Autodesk Inventor part; units mm, degrees
ref_plane "YZ Plane" through (0, 0, 0) normal (1, 0, 0) x (0, 1, 0)
ref_plane "XZ Plane" through (0, 0, 0) normal (0, 1, 0) x (-1, 0, 0)
ref_plane "XY Plane" through (0, 0, 0) normal (0, 0, 1) x (1, 0, 0)
sketch "Sketch1" plane through (0, 0, 0) normal (0, 0, 1) x (1, 0, 0)
  line L0 (0, 0) -> (44, 0)
  line L1 (44, 0) -> (44, 10)
  line L2 (44, 10) -> (0, 10)
  line L3 (0, 10) -> (0, 0)
  circle A0 centre (29.5, 5) radius 2.25
  circle A1 centre (14.5, 5) radius 2.25
  line L4 (14.5, 5) -> (29.5, 5) construction
  point P0 (0, 5)
  point P1 (22, 5)
  point P2 (22, 10)
  dimension "d0" = 10
  dimension "d1" = 44
  dimension "d2" = 4.5
  dimension "d13" = 4.5
  dimension "d14" = 15
extrude "Extrusion3" add sketch "Sketch1" along normal blind 6
sketch "Sketch3" plane through (0, 0, 6) normal (0, 0, 1) x (1, 0, 0)
  line L0 (0, 0) -> (44, 0)
  line L1 (44, 10) -> (0, 10)
  line L2 (6.5, 10) -> (14.5, 10)
  line L3 (14.5, 10) -> (14.5, 14)
  line L4 (12.5, 16) -> (8.5, 16)
  line L5 (6.5, 14) -> (6.5, 10)
  line L6 (29.5, 10) -> (37.5, 10)
  line L7 (37.5, 10) -> (37.5, 14)
  line L8 (35.5, 16) -> (31.5, 16)
  line L9 (29.5, 14) -> (29.5, 10)
  line L10 (6.5, 0) -> (14.5, 0)
  line L11 (14.5, 0) -> (14.5, -4)
  line L12 (12.5, -6) -> (8.5, -6)
  line L13 (6.5, -4) -> (6.5, 0)
  line L14 (29.5, 0) -> (37.5, 0)
  line L15 (37.5, 0) -> (37.5, -4)
  line L16 (35.5, -6) -> (31.5, -6)
  line L17 (29.5, -4) -> (29.5, 0)
  arc A0 (8.5, 16) -> (6.5, 14) centre (8.5, 14) ccw
  arc A1 (14.5, 14) -> (12.5, 16) centre (12.5, 14) ccw
  arc A2 (31.5, 16) -> (29.5, 14) centre (31.5, 14) ccw
  arc A3 (37.5, 14) -> (35.5, 16) centre (35.5, 14) ccw
  arc A4 (6.5, -4) -> (8.5, -6) centre (8.5, -4) ccw
  arc A5 (12.5, -6) -> (14.5, -4) centre (12.5, -4) ccw
  arc A6 (29.5, -4) -> (31.5, -6) centre (31.5, -4) ccw
  arc A7 (35.5, -6) -> (37.5, -4) centre (35.5, -4) ccw
  line L18 (14.5, 12.5251) -> (29.5, 12.5251) construction
  point P0 (22, 12.5251)
  point P1 (22, 10)
  dimension "d17" = 2
  dimension "d18" = 8
  dimension "d19" = 8
  dimension "d20" = 6
  dimension "d21" = 6
  dimension "d22" = 15
extrude "Extrusion4" add sketch "Sketch3" against normal blind 6
properties part number "y_carriage_belt_mount_bed_holder"
Can you work these out from the model? Positions are in its coordinate system, mm. A direction names the side the tool comes from. Give positions to 0.01 mm unless a question says otherwise; leave off trailing zeros. Loops run counter-clockwise (first coordinate to the right, second up) from the corner with the lowest first, then second, coordinate; pieces in that order, holes last. Notation, with made-up numbers: (89.25, 66.5) -> (120.25, 66.5) arc R18 cw to (120.25, 101.5) -> close; hole circle Ø8 at (-34, -38.5). An arc over 180 degrees is marked (long way). Return JSON: item names as keys, results as strings.
Q1. For pin 1 Ø1.8 at (x, z) = (40.5, 3) entering from -Y; pin 2 Ø2 at (y, z) = (-3, 2.5) entering from -X; pin 3 Ø6 at (x, y) = (14.5, 5) entering from +Z; pin 4 Ø1.8 at (x, z) = (21, 2.5) entering from +Y, each with a flat end and sliding along its axis, tell me the tip position at first contact or that it passes through.
Checks:
{"pin 1": "stops at y = 0", "pin 2": "stops at x = 6.5", "pin 3": "stops at z = 6", "pin 4": "stops at y = 10"}
Q2. On a 3-axis mill with a long thin cutter (end or side, diameter ignored), from which of +Z, -Z, +X, -X, +Y, -Y can I reach the whole of each face in a straight line? I mean faces 4 (the face through (6.5, -2, 3)), 5 (the face through (37.5, 12, 3)), 6 (the face through (22, 10, 3)), 7 (the face through (30.07, -5.4, 3.04)). Say none if no direction works.
Checks:
{"face 4": "+Z, -Z, -X, -Y", "face 5": "+Z, -Z, +X, +Y", "face 6": "+Z, -Z, +Y", "face 7": "+Z, -Z, -Y"}
Q3. I want a section at B-B, the plane z = 4.35. Count the separate pieces of the cut face and the enclosed holes in it, then the cut area to 3 significant figures.
Checks:
{"separate pieces": "1", "enclosed holes": "2", "area": "593 mm2"}
Q4. We'd pull the mould along X, two halves only. Please class faces 1 (the face through (37.5, -2, 3)), 2 (the face through (11, 16, 3)), 3 (the face through (16.646, 4.324, 2.958)): released by +X, released by -X, zero draft, split by the parting line, or undercut.
Checks:
{"face 1": "released by +X", "face 2": "zero draft", "face 3": "undercut"}
Q5. I need wall thicknesses on probe 1 along X at (y, z) = (3.25, 0.85); probe 2 along X at (y, z) = (11, 1.85); probe 3 along X at (y, z) = (14.75, 0.7). Which ranges of each line are inside material? Lowest first, please.
Checks:
{"probe 1": "x = 0 to 13.09, 15.91 to 28.09, 30.91 to 44", "probe 2": "x = 6.5 to 14.5, 29.5 to 37.5", "probe 3": "x = 6.65 to 14.35, 29.65 to 37.35"}
Q6. I want a section at C-C, the plane y = 10.75. List the corners of the cut face in (x, z) for me.
Checks:
{"outline": "(6.5, 0) -> (14.5, 0) -> (14.5, 6) -> (6.5, 6) -> close; (29.5, 0) -> (37.5, 0) -> (37.5, 6) -> (29.5, 6) -> close"}
Q7. I want a section at D-D, the plane x = 18. List the corners of the cut face in (y, z) for me.
Checks:
{"outline": "(0, 0) -> (10, 0) -> (10, 6) -> (0, 6) -> close"}
Q8. I want a section at A-A, the plane y = 5. List the corners of the cut face in (x, z) for me.
Checks:
{"outline": "(0, 0) -> (12.25, 0) -> (12.25, 6) -> (0, 6) -> close; (16.75, 0) -> (27.25, 0) -> (27.25, 6) -> (16.75, 6) -> close; (31.75, 0) -> (44, 0) -> (44, 6) -> (31.75, 6) -> close"}
